Source: three-view drawing plus pictorial views. Frame: mm from the lowest corner of the part. A direction names the side the tool comes from. Give positions to 0.01 mm unless a question says otherwise; leave off trailing zeros. Write each loop counter-clockwise with the first axis right and the second up, starting at its lowest first coordinate (ties: lowest second). Pieces come first, ordered by that corner, then holes.
Q1. Reachability of the marked faces 4, 5, 6, 7 and 8 from +Z, -Z, +X, -X, +Y, -Y: full face, straight path, thin tool, end or side. Return the list, or none.
Q2. Cut plane D-D on y = 3. Return the cut outline in (x, z), plus the area to 3 significant figures.
Q3. Pin query (flat end, axial travel): pin 1 (0.9 mm diameter, centred on x = 6.5, y = 2.5, fed in from -Z); pin 2 (0.9 mm diameter, centred on x = 20, y = 2, fed in from -Z); pin 3 (1.5 mm diameter, centred on y = 2.5, z = 1.5, fed in from +X); pin 4 (1.5 mm diameter, centred on x = 19.5, y = 0.5, fed in from +Z). Return the tip coordinate at first contact, or that it passes through.
Q4. Cut plane C-C on z = 6.5. Return the cut outline in (x, y), plus the area to 3 significant figures.
Q5. Draft query along Z for the marked faces 1, 2 and 3. Return one class per face: pulls with the +Z half, pulls with the -Z half, needs draft (parallel to the pull), parting line crosses it, or undercut.
Q6. Line query: L1, parallel to Z at x = 4, y = 1.55; L2, parallel to X at y = 2.3, z = 5.75; L3, parallel to Z at x = 16.5, y = 3. Output: solid intervals per line, ascending.
Q7. Cut plane B-B on y = 0.5. Return the cut outline in (x, z), plus the area to 3 significant figures.
Q8. Cut plane A-A on x = 10.25. Return the cut outline in (y, z).
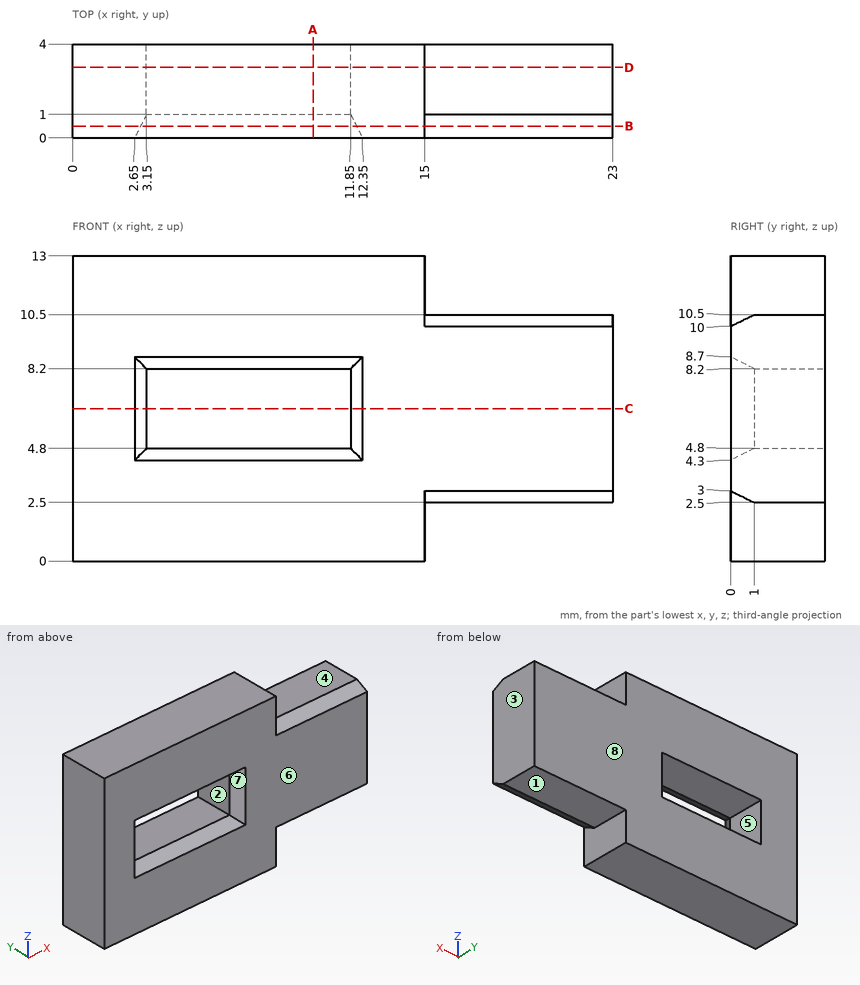
Data:
1. face 4: +Z, +X, +Y, -Y
1. face 5: +Y, -Y
1. face 6: +Z, -Z, +X, -X, -Y
1. face 7: -Y
1. face 8: +Z, -Z, +X, -X, +Y
2. outline: (0, 0) - (15, 0) - (15, 2.5) - (23, 2.5) - (23, 10.5) - (15, 10.5) - (15, 13) - (0, 13) - close; hole (3.15, 4.8) - (11.85, 4.8) - (11.85, 8.2) - (3.15, 8.2) - close
2. area: 229 mm2
3. pin 1: stops at z = 0
3. pin 2: stops at z = 2.5
3. pin 3: stops at x = 15
3. pin 4: stops at z = 10.5
4. outline: (0, 0) - (2.65, 0) - (3.15, 1) - (3.15, 4) - (0, 4) - close; (11.85, 1) - (12.35, 0) - (23, 0) - (23, 4) - (11.85, 4) - close
4. area: 56.7 mm2
5. face 1: pulls with the -Z half
5. face 2: undercut
5. face 3: needs draft
6. L1: z = 0 to 4.8, 8.2 to 13
6. L2: x = 0 to 3.15, 11.85 to 23
6. L3: z = 2.5 to 10.5
7. outline: (0, 0) - (15, 0) - (15, 2.75) - (23, 2.75) - (23, 10.25) - (15, 10.25) - (15, 13) - (0, 13) - close; hole (2.9, 4.55) - (12.1, 4.55) - (12.1, 8.45) - (2.9, 8.45) - close
7. area: 219 mm2
8. outline: (0, 0) - (4, 0) - (4, 4.8) - (1, 4.8) - (0, 4.3) - close; (0, 8.7) - (1, 8.2) - (4, 8.2) - (4, 13) - (0, 13) - close
